Build history of the part. All positions in model axes, mm. Give positions to 0.01 mm unless a question says otherwise; leave off trailing zeros. Order: outer loops, then holes, each group sorted by start corner. A loop starts at its lowest first (then second) coordinate and runs counter-clockwise, first axis right, second up. Notation, with made-up numbers: M 40.25,-10.75 L 56.25,-10.75 A25 ccw 56.25,26.25 Z; hole C 60.5,-30.75 d11. An arc over 180 degrees is marked long. One line per item, written item: value.
from build123d import *

# Parameters (mm, degrees)
F0_W          = 14.1733624041
F0_H          = 41.7313948274
F1_DEPTH      = 25.4
F2_R          = 5.08
F3_R          = 5.08
F4_R          = 5.08
F5_R          = 5.08
F6_W          = 31.9113396108
F6_H          = 17.5824901089
F7_DEPTH      = 12.7
F8_DEPTH      = 25.4
F10_D         = 6.35
F11_D         = 6.35
F12_T1_DEPTH  = 15.24
F12_T3_DEPTH  = 31.5713948274
F12_T6_ANGLE  = 90
F12_T8_ANGLE  = 90
F12_T10_ANGLE = 90
F12_T12_ANGLE = 90
F12_T14_ANGLE = 90
F12_T18_DEPTH = 31.5713948274
F12_T24_DEPTH = 31.5713948274
F12_T30_DEPTH = 31.5713948274
F12_T36_ANGLE = 90
F12_T42_ANGLE = 90
F12_T48_ANGLE = 90
F12_T54_DEPTH = 15.24
F12_T59_ANGLE = 90
F12_T65_ANGLE = 90
F12_T71_ANGLE = 90
F12_T77_DEPTH = 31.5713948274
F12_T83_DEPTH = 31.5713948274
F12_T89_DEPTH = 31.5713948274
F12_T93_ANGLE = 90


# Not quite as in the source:
# - a fillet or chamfer that OpenCascade refuses, or shapes differently, is made with other operations: its cross-section is extruded or revolved along the edge and cut away or added


with BuildPart() as f1:
    # F0 (on Top) → F1 (new body)
    with BuildSketch(Plane.XY):
        with Locations((-43.3002728969, -20.8656974137)):
            Rectangle(F0_W, F0_H)
    extrude(amount=F1_DEPTH)

    # F2
    f2_edges = [f1.edges().sort_by_distance(p)[0] for p in [
        (-43.300273, -41.731395, 25.4),
    ]]
    fillet(f2_edges, radius=F2_R)

    # F3
    f3_edges = [f1.edges().sort_by_distance(p)[0] for p in [
        (-43.300273, -41.731395, 0),
    ]]
    fillet(f3_edges, radius=F3_R)

    # F4
    f4_edges = [f1.edges().sort_by_distance(p)[0] for p in [
        (-43.300273, 0, 0),
    ]]
    fillet(f4_edges, radius=F4_R)

    # F5
    f5_edges = [f1.edges().sort_by_distance(p)[0] for p in [
        (-43.300273, 0, 25.4),
    ]]
    fillet(f5_edges, radius=F5_R)

    # F1_face (on face) + F6 (on face) → F7 (join)
    with BuildSketch(Plane(origin=(-50.3869540989, -20.8656974137, 12.7), x_dir=(0, -1, 0), z_dir=(-1, 0, 0))):
        with BuildLine():
            Line((-20.8656974137, 7.62), (-20.8656974137, -7.62))
            ThreePointArc((-20.8656974137, -7.62), (-19.3777998621, -11.2121024484), (-15.7856974137, -12.7))
            Line((-15.7856974137, -12.7), (15.7856974137, -12.7))
            ThreePointArc((15.7856974137, -12.7), (19.3777998621, -11.2121024484), (20.8656974137, -7.62))
            Line((20.8656974137, -7.62), (20.8656974137, 7.62))
            ThreePointArc((20.8656974137, 7.62), (19.3777998621, 11.2121024484), (15.7856974137, 12.7))
            Line((15.7856974137, 12.7), (-15.7856974137, 12.7))
            ThreePointArc((-15.7856974137, 12.7), (-19.3777998621, 11.2121024484), (-20.8656974137, 7.62))
        make_face()
    with BuildSketch(Plane(origin=(-50.3869540989, 0, 0), x_dir=(0, -1, 0), z_dir=(-1, 0, 0))):
        with Locations((18.8954193145, 13.6700686999)):
            Rectangle(F6_W, F6_H)
    extrude(amount=-F7_DEPTH)

    # F6 (on face) → F8 (join)
    with BuildSketch(Plane(origin=(-50.3869540989, 0, 0), x_dir=(0, -1, 0), z_dir=(-1, 0, 0))):
        with Locations((18.8954193145, 13.6700686999)):
            Rectangle(F6_W, F6_H)
    extrude(amount=F8_DEPTH)

    # F10 (through all)
    with Locations(Plane.XY.offset(22.4613137543)):
        with Locations((-71.6206654906, -29.537204653)):
            Hole(F10_D / 2)

    # F11 (through all)
    with Locations(Plane.XY.offset(22.4613137543)):
        with Locations((-72.0812156796, -7.7047413215)):
            Hole(F11_D / 2)

    # F12: chamfer of 5.08 on 4 edges, made by hand

    # F12_s2 → F12_t1 (cut)
    with BuildSketch(Plane.XY.offset(5.08)):
        Polygon((-36.2135916948, -36.6513948274), (-41.2935916948, -41.7313948274), (-36.2135916948, -41.7313948274), align=None)
        Polygon((-41.2935916948, 0), (-36.2135916948, -5.08), (-36.2135916948, 0), align=None)
        Polygon((-50.3869540989, -36.6513948274), (-45.3069540989, -41.7313948274), (-50.3869540989, -41.7313948274), align=None)
    extrude(amount=F12_T1_DEPTH, mode=Mode.SUBTRACT)

    # F12_s4 → F12_t3 (cut)
    with BuildSketch(Plane.XZ.offset(5.08)):
        Polygon((-36.2135916948, 20.32), (-41.2935916948, 25.4), (-36.2135916948, 25.4), align=None)
        Polygon((-36.2135916948, 5.08), (-41.2935916948, 0), (-36.2135916948, 0), align=None)
    extrude(amount=F12_T3_DEPTH, mode=Mode.SUBTRACT)

    # F12_s5 → F12_t6 (revolve, cut)
    with BuildSketch(Plane.XY.offset(20.32)):
        Polygon((-50.3869540989, -36.6513948274), (-45.3069540989, -41.7313948274), (-50.3869540989, -41.7313948274), align=None)
    revolve(axis=Axis((-50.3869540989, -36.6513948274, 20.32), (-1, 0, 0)), revolution_arc=F12_T6_ANGLE, mode=Mode.SUBTRACT)

    # F12_s7 → F12_t8 (revolve, cut)
    with BuildSketch(Plane.XY.offset(20.32)):
        Polygon((-36.2135916948, -36.6513948274), (-41.2935916948, -41.7313948274), (-36.2135916948, -41.7313948274), align=None)
    revolve(axis=Axis((-36.2135916948, -36.6513948274, 20.32), (-1, 0, 0)), revolution_arc=F12_T8_ANGLE, mode=Mode.SUBTRACT)

    # F12_s9 → F12_t10 (revolve, cut)
    with BuildSketch(Plane.XY.offset(20.32)):
        Polygon((-36.2135916948, -5.08), (-41.2935916948, 0), (-36.2135916948, 0), align=None)
    revolve(axis=Axis((-36.2135916948, -5.08, 20.32), (1, 0, 0)), revolution_arc=F12_T10_ANGLE, mode=Mode.SUBTRACT)

    # F12_s11 → F12_t12 (revolve, cut)
    with BuildSketch(Plane.XZ.offset(5.08)):
        Polygon((-41.2935916948, 0), (-36.2135916948, 5.08), (-36.2135916948, 0), align=None)
    revolve(axis=Axis((-36.2135916948, -5.08, 5.08), (1, 0, 0)), revolution_arc=F12_T12_ANGLE, mode=Mode.SUBTRACT)

    # F12_s13 → F12_t14 (revolve, cut)
    with BuildSketch(Plane.XY.offset(5.08)):
        Polygon((-36.2135916948, -36.6513948274), (-41.2935916948, -41.7313948274), (-36.2135916948, -41.7313948274), align=None)
    revolve(axis=Axis((-36.2135916948, -36.6513948274, 5.08), (1, 0, 0)), revolution_arc=F12_T14_ANGLE, mode=Mode.SUBTRACT)


with BuildPart() as f12_tool16:
    # F12_s17 → F12_t18 (new body)
    with BuildSketch(Plane.XZ.offset(5.08)):
        Polygon((-50.3869540989, 20.32), (-45.3069540989, 25.4), (-50.3869540989, 25.4), align=None)
    extrude(amount=F12_T18_DEPTH)

    split(bisect_by=Plane.XY.offset(22.4613137543), keep=Keep.TOP)

    split(bisect_by=Plane.XZ.offset(34.8510891199), keep=Keep.BOTTOM)


with BuildPart() as f1_1:
    add(f1.part)

    # F12_t15: cut F12_tool16
    add(f12_tool16.part, mode=Mode.SUBTRACT)


with BuildPart() as f12_tool22:
    # F12_s23 → F12_t24 (new body)
    with BuildSketch(Plane.XZ.offset(5.08)):
        Polygon((-50.3869540989, 20.32), (-45.3069540989, 25.4), (-50.3869540989, 25.4), align=None)
    extrude(amount=F12_T24_DEPTH)

    split(bisect_by=Plane.XY.offset(22.4613137543), keep=Keep.BOTTOM)

    split(bisect_by=Plane.XZ.offset(34.8510891199), keep=Keep.TOP)


with BuildPart() as f1_2:
    add(f1_1.part)

    # F12_t21: cut F12_tool22
    add(f12_tool22.part, mode=Mode.SUBTRACT)


with BuildPart() as f12_tool28:
    # F12_s29 → F12_t30 (new body)
    with BuildSketch(Plane.XZ.offset(5.08)):
        Polygon((-50.3869540989, 20.32), (-45.3069540989, 25.4), (-50.3869540989, 25.4), align=None)
    extrude(amount=F12_T30_DEPTH)

    split(bisect_by=Plane.XY.offset(22.4613137543), keep=Keep.TOP)

    split(bisect_by=Plane.XZ.offset(34.8510891199), keep=Keep.TOP)


with BuildPart() as f1_3:
    add(f1_2.part)

    # F12_t27: cut F12_tool28
    add(f12_tool28.part, mode=Mode.SUBTRACT)


with BuildPart() as f12_tool34:
    # F12_s35 → F12_t36 (revolve)
    with BuildSketch(Plane.XY.offset(20.32)):
        Polygon((-45.3069540989, 0), (-50.3869540989, -5.08), (-50.3869540989, 0), align=None)
    revolve(axis=Axis((-50.3869540989, -5.08, 20.32), (1, 0, 0)), revolution_arc=F12_T36_ANGLE)

    split(bisect_by=Plane.XZ.offset(2.9397495091), keep=Keep.BOTTOM)

    split(bisect_by=Plane.XY.offset(22.4613137543), keep=Keep.BOTTOM)


with BuildPart() as f1_4:
    add(f1_3.part)

    # F12_t33: cut F12_tool34
    add(f12_tool34.part, mode=Mode.SUBTRACT)


with BuildPart() as f12_tool40:
    # F12_s41 → F12_t42 (revolve)
    with BuildSketch(Plane.XY.offset(20.32)):
        Polygon((-45.3069540989, 0), (-50.3869540989, -5.08), (-50.3869540989, 0), align=None)
    revolve(axis=Axis((-50.3869540989, -5.08, 20.32), (1, 0, 0)), revolution_arc=F12_T42_ANGLE)

    split(bisect_by=Plane.XZ.offset(2.9397495091), keep=Keep.BOTTOM)

    split(bisect_by=Plane.XY.offset(22.4613137543), keep=Keep.TOP)


with BuildPart() as f1_5:
    add(f1_4.part)

    # F12_t39: cut F12_tool40
    add(f12_tool40.part, mode=Mode.SUBTRACT)


with BuildPart() as f12_tool46:
    # F12_s47 → F12_t48 (revolve)
    with BuildSketch(Plane.XY.offset(20.32)):
        Polygon((-45.3069540989, 0), (-50.3869540989, -5.08), (-50.3869540989, 0), align=None)
    revolve(axis=Axis((-50.3869540989, -5.08, 20.32), (1, 0, 0)), revolution_arc=F12_T48_ANGLE)

    split(bisect_by=Plane.XZ.offset(2.9397495091), keep=Keep.TOP)

    split(bisect_by=Plane.XY.offset(22.4613137543), keep=Keep.TOP)


with BuildPart() as f1_6:
    add(f1_5.part)

    # F12_t45: cut F12_tool46
    add(f12_tool46.part, mode=Mode.SUBTRACT)


with BuildPart() as f12_tool52:
    # F12_s53 → F12_t54 (new body)
    with BuildSketch(Plane.XY.offset(5.08)):
        Polygon((-45.3069540989, 0), (-50.3869540989, -5.08), (-50.3869540989, 0), align=None)
    extrude(amount=F12_T54_DEPTH)

    split(bisect_by=Plane.XZ.offset(2.9397495091), keep=Keep.BOTTOM)


with BuildPart() as f1_7:
    add(f1_6.part)

    # F12_t51: cut F12_tool52
    add(f12_tool52.part, mode=Mode.SUBTRACT)


with BuildPart() as f12_tool57:
    # F12_s58 → F12_t59 (revolve)
    with BuildSketch(Plane.XZ.offset(5.08)):
        Polygon((-45.3069540989, 0), (-50.3869540989, 5.08), (-50.3869540989, 0), align=None)
    revolve(axis=Axis((-50.3869540989, -5.08, 5.08), (1, 0, 0)), revolution_arc=F12_T59_ANGLE)

    split(bisect_by=Plane.XZ.offset(2.9397495091), keep=Keep.TOP)

    split(bisect_by=Plane.XY.offset(4.8788236454), keep=Keep.BOTTOM)


with BuildPart() as f1_8:
    add(f1_7.part)

    # F12_t56: cut F12_tool57
    add(f12_tool57.part, mode=Mode.SUBTRACT)


with BuildPart() as f12_tool63:
    # F12_s64 → F12_t65 (revolve)
    with BuildSketch(Plane.XZ.offset(5.08)):
        Polygon((-45.3069540989, 0), (-50.3869540989, 5.08), (-50.3869540989, 0), align=None)
    revolve(axis=Axis((-50.3869540989, -5.08, 5.08), (1, 0, 0)), revolution_arc=F12_T65_ANGLE)

    split(bisect_by=Plane.XZ.offset(2.9397495091), keep=Keep.BOTTOM)

    split(bisect_by=Plane.XY.offset(4.8788236454), keep=Keep.BOTTOM)


with BuildPart() as f1_9:
    add(f1_8.part)

    # F12_t62: cut F12_tool63
    add(f12_tool63.part, mode=Mode.SUBTRACT)


with BuildPart() as f12_tool69:
    # F12_s70 → F12_t71 (revolve)
    with BuildSketch(Plane.XZ.offset(5.08)):
        Polygon((-45.3069540989, 0), (-50.3869540989, 5.08), (-50.3869540989, 0), align=None)
    revolve(axis=Axis((-50.3869540989, -5.08, 5.08), (1, 0, 0)), revolution_arc=F12_T71_ANGLE)

    split(bisect_by=Plane.XZ.offset(2.9397495091), keep=Keep.BOTTOM)

    split(bisect_by=Plane.XY.offset(4.8788236454), keep=Keep.TOP)


with BuildPart() as f1_10:
    add(f1_9.part)

    # F12_t68: cut F12_tool69
    add(f12_tool69.part, mode=Mode.SUBTRACT)


with BuildPart() as f12_tool75:
    # F12_s76 → F12_t77 (new body)
    with BuildSketch(Plane.XZ.offset(5.08)):
        Polygon((-50.3869540989, 5.08), (-45.3069540989, 0), (-50.3869540989, 0), align=None)
    extrude(amount=F12_T77_DEPTH)

    split(bisect_by=Plane.XZ.offset(34.8510891199), keep=Keep.BOTTOM)

    split(bisect_by=Plane.XY.offset(4.8788236454), keep=Keep.BOTTOM)


with BuildPart() as f1_11:
    add(f1_10.part)

    # F12_t74: cut F12_tool75
    add(f12_tool75.part, mode=Mode.SUBTRACT)


with BuildPart() as f12_tool81:
    # F12_s82 → F12_t83 (new body)
    with BuildSketch(Plane.XZ.offset(5.08)):
        Polygon((-50.3869540989, 5.08), (-45.3069540989, 0), (-50.3869540989, 0), align=None)
    extrude(amount=F12_T83_DEPTH)

    split(bisect_by=Plane.XZ.offset(34.8510891199), keep=Keep.TOP)

    split(bisect_by=Plane.XY.offset(4.8788236454), keep=Keep.TOP)


with BuildPart() as f1_12:
    add(f1_11.part)

    # F12_t80: cut F12_tool81
    add(f12_tool81.part, mode=Mode.SUBTRACT)


with BuildPart() as f12_tool87:
    # F12_s88 → F12_t89 (new body)
    with BuildSketch(Plane.XZ.offset(5.08)):
        Polygon((-50.3869540989, 5.08), (-45.3069540989, 0), (-50.3869540989, 0), align=None)
    extrude(amount=F12_T89_DEPTH)

    split(bisect_by=Plane.XZ.offset(34.8510891199), keep=Keep.TOP)

    split(bisect_by=Plane.XY.offset(4.8788236454), keep=Keep.BOTTOM)


with BuildPart() as f1_13:
    add(f1_12.part)

    # F12_t86: cut F12_tool87
    add(f12_tool87.part, mode=Mode.SUBTRACT)

    # F12_s92 → F12_t93 (revolve, cut)
    with BuildSketch(Plane.XY.offset(5.08)):
        Polygon((-50.3869540989, -36.6513948274), (-45.3069540989, -41.7313948274), (-50.3869540989, -41.7313948274), align=None)
    revolve(axis=Axis((-50.3869540989, -36.6513948274, 5.08), (1, 0, 0)), revolution_arc=F12_T93_ANGLE, mode=Mode.SUBTRACT)


solid = f1_13.part
1) Saw through at B-B, the plane z = 6.5. Write the cut outline in (x, y) (3 decimals), then the cut area to 3 significant figures.
Check values:
outline: M -75.787,-34.851 L -50.387,-34.851 L -50.387,-36.651 L -45.307,-41.731 L -41.294,-41.731 L -36.214,-36.651 L -36.214,-5.08 L -41.294,0 L -45.307,0 L -48.247,-2.94 L -75.787,-2.94 Z; hole C -72.081,-7.705 d6.35; hole C -71.621,-29.537 d6.35
area: 1,290 mm^2
2) Saw through at A-A, the plane y = -25. Write the cut outline in (x, z), then the cut area to 3 significant figures.
Check values:
outline: M -75.79,4.88 L -50.19,4.88 L -45.31,0 L -41.29,0 L -36.21,5.08 L -36.21,20.32 L -41.29,25.4 L -45.31,25.4 L -48.25,22.46 L -75.79,22.46 Z
area: 757 mm^2
3) Saw through at C-C, the plane x = -44.5. Write the cut outline in (y, z).
Check values:
outline: M -41.73,5.08 A5.08 ccw -36.65,0 L -5.08,0 A5.08 ccw 0,5.08 L 0,20.32 A5.08 ccw -5.08,25.4 L -36.65,25.4 A5.08 ccw -41.73,20.32 Z
4) Drill centre lines: probe 1 along Y at (x, z) = (-74, 9.5); probe 2 along Y at (x, z) = (-54.5, 10.75); probe 3 along Z at (x, y) = (-65, -3.5). Where is each one in solid material? Low to high. Write a range as from..to.
Check values:
probe 1: -34.85..-31.64, -27.43..-10.23, -5.18..-2.94
probe 2: -34.85..-2.94
probe 3: 4.88..22.46
5) Pin check, flat tips, straight feed: pin 1 (0.5 mm diameter, centred on y = -36, z = 10, fed in from -X); pin 2 (7.5 mm diameter, centred on x = -71.62, y = -29.54, fed in from -Z); pin 3 (14 mm diameter, centred on x = -59.5, z = 11.5, fed in from -Y). Stop position of each tip, or through.
Check values:
pin 1: x = -50.39
pin 2: z = 4.88
pin 3: y = -34.85
6) Saw through at D-D, the plane x = -66.5. Write the cut outline in (y, z).
Check values:
outline: M -34.85,4.88 L -2.94,4.88 L -2.94,22.46 L -34.85,22.46 Z
7) Mould opens along Y. For faces 1 (the face through (-62, -34.851, 14)), 2 (the face through (-75.787, -19, 14)), 3 (the face through (-46.797, -2.514, 22.83)), 4 (the face through (-74.554, -30.753, 13.547)) say: released by +Y, released by -Y, zero draft, split by the parting line, or undercut.
Check values:
face 1: released by -Y
face 2: zero draft
face 3: released by +Y
face 4: undercut
